Input: part model. Units: mm. Frame: model coordinates. Give positions to 0.01 mm unless a question says otherwise; leave off trailing zeros. Write each loop counter-clockwise with the first axis right and the second up, starting at its lowest first coordinate (ties: lowest second). Pieces come first, ordered by that corner, then holes. Notation, with made-up numbers: (68.5, -9) - (73.5, -9) arc R16 cw to (73.5, 18) - close; hole circle Ø1 at (2.25, 64.25). An arc over 180 degrees is marked (long way). Use a Markdown table: item, result. Add a question column.
1. Section query A-A, the plane z = 0. Return loops of the section in (x, y), plus the area to 4 significant figures.
2. Mould query, pull axis Z, two halves, no side actions, for faces 1 (the flat face through (-6, -41, 0)), 2 (the flat face through (13.421, -20.213, 6.456)). Classes: released by +Z, released by -Z, zero draft, split by the parting line, or undercut.
3. Section query D-D, the plane z = -15. Return loops of the section in (x, y), plus the area to 3 significant figures.
4. Material intervals for probe 1 along Z at (x, y) = (8.5, -7); probe 2 along X at (y, z) = (-26, 10.5); probe 3 along X at (y, z) = (-26, -19), sorted ascending.
5. Section query B-B, the plane x = 0. Return loops of the section in (y, z).
6. Pin query (flat end, axial travel): pin 1 (5 mm diameter, centred on y = -17, z = -12, fed in from +X); pin 2 (8 mm diameter, centred on x = 20, y = -30, fed in from -Z); pin 3 (12 mm diameter, centred on x = 4.5, y = -5.5, fed in from -Z). Return the tip coordinate at first contact, or that it passes through.
7. Section query C-C, the plane y = -8.5. Count the separate pieces of the cut face and the enclosed holes in it, plus the area to 3 significant figures.
```python
from build123d import *

# Parameters (mm, degrees)
F0_R     = 26.25
F1_DEPTH = 41


with BuildPart() as f1:
    # F0 (on Front) → F1 (new body)
    with BuildSketch(Plane.XZ):
        Circle(F0_R)
        with BuildLine():
            ThreePointArc((-1.5, -22.449944), (-11.250362, -19.485363), (-18.692687, -12.523316))
            Line((-18.692687, -12.523316), (-6.088184, -4.379957))
            ThreePointArc((-6.088184, -4.379957), (-3.75, -6.495191), (-0.749062, -7.4625))
            Line((-0.749062, -7.4625), (-1.5, -22.449944))
        make_face(mode=Mode.SUBTRACT)
        with BuildLine():
            ThreePointArc((18.692222, -12.52401), (11.249638, -19.48578), (1.499166, -22.45))
            Line((1.499166, -22.45), (0.749062, -7.4625))
            ThreePointArc((0.749062, -7.4625), (3.75, -6.495191), (6.088184, -4.379957))
            Line((6.088184, -4.379957), (18.692222, -12.52401))
        make_face(mode=Mode.SUBTRACT)
        with BuildLine():
            ThreePointArc((20.192222, 9.925934), (22.5, -0.000418), (20.191854, -9.926684))
            Line((20.191854, -9.926684), (6.837246, -3.082543))
            ThreePointArc((6.837246, -3.082543), (7.5, 0), (6.837246, 3.082543))
            Line((6.837246, 3.082543), (20.192222, 9.925934))
        make_face(mode=Mode.SUBTRACT)
        with BuildLine():
            ThreePointArc((-20.192222, -9.925934), (-22.5, 0.000418), (-20.191854, 9.926684))
            Line((-20.191854, 9.926684), (-6.837246, 3.082543))
            ThreePointArc((-6.837246, 3.082543), (-7.5, 0), (-6.837246, -3.082543))
            Line((-6.837246, -3.082543), (-20.192222, -9.925934))
        make_face(mode=Mode.SUBTRACT)
        with BuildLine():
            ThreePointArc((-18.692222, 12.52401), (-11.249638, 19.48578), (-1.499166, 22.45))
            Line((-1.499166, 22.45), (-0.749062, 7.4625))
            ThreePointArc((-0.749062, 7.4625), (-1.737374, 7.295994), (-2.69466, 6.9992))
            ThreePointArc((-2.69466, 6.9992), (-3.75, 6.495191), (-4.714155, 5.833245))
            ThreePointArc((-4.714155, 5.833245), (-5.44983, 5.152607), (-6.088184, 4.379957))
            Line((-6.088184, 4.379957), (-18.692222, 12.52401))
        make_face(mode=Mode.SUBTRACT)
        with BuildLine():
            ThreePointArc((-2.148919, 5.06282), (2.772797, -4.749905), (-3.352022, 4.360498))
            ThreePointArc((-3.352022, 4.360498), (-2.772797, 4.749905), (-2.148919, 5.06282))
        make_face(mode=Mode.SUBTRACT)
        with BuildLine():
            Line((0.749062, 7.4625), (1.5, 22.449944))
            ThreePointArc((1.5, 22.449944), (11.250362, 19.485363), (18.692687, 12.523316))
            Line((18.692687, 12.523316), (6.088184, 4.379957))
            ThreePointArc((6.088184, 4.379957), (3.75, 6.495191), (0.749062, 7.4625))
        make_face(mode=Mode.SUBTRACT)
    extrude(amount=F1_DEPTH)


solid = f1.part
```
Result sheet:
| question | item | result |
|---|---|---|
| 1 | outline | (-26.25, -41) - (-22.5, -41) - (-22.5, 0) - (-26.25, 0) - close; (-7.5, -41) - (-5.5, -41) - (-5.5, 0) - (-7.5, 0) - close; (5.5, -41) - (7.5, -41) - (7.5, 0) - (5.5, 0) - close; (22.5, -41) - (26.25, -41) - (26.25, 0) - (22.5, 0) - close |
| 1 | area | 471.5 mm² |
| 2 | face 1 | zero draft |
| 2 | face 2 | undercut |
| 3 | outline | (-21.54, -41) - (-16.77, -41) - (-16.77, 0) - (-21.54, 0) - close; (-1.13, -41) - (1.13, -41) - (1.13, 0) - (-1.13, 0) - close; (16.77, -41) - (21.54, -41) - (21.54, 0) - (16.77, 0) - close |
| 3 | area | 484 mm² |
| 4 | probe 1 | z = -24.84 to -20.83, -5.94 to -3.93, 3.93 to 5.94, 20.83 to 24.84 |
| 4 | probe 2 | x = -24.06 to -15.56, -0.9 to 0.9, 15.56 to 24.06 |
| 4 | probe 3 | x = -18.11 to -12.05, -1.33 to 1.33, 12.05 to 18.11 |
| 5 | outline | (-41, -26.25) - (0, -26.25) - (0, -5.5) - (-41, -5.5) - close; (-41, 5.5) - (0, 5.5) - (0, 26.25) - (-41, 26.25) - close |
| 6 | pin 1 | stops at x = 24.47 |
| 6 | pin 2 | stops at z = -20.81 |
| 6 | pin 3 | stops at z = -26.25 |
| 7 | separate pieces | 1 |
| 7 | enclosed holes | 7 |
| 7 | area | 859 mm² |
